```python
from build123d import *

# Parameters (mm, degrees)
SKETCH_1_W             = 56
SKETCH_1_H             = 54
EXTRUDE_492_DEPTH      = 12.5
SKETCH_3_W             = 36
SKETCH_3_H             = 46
CUT_EXTRUDE_735_DEPTH  = 41.856456038
SKETCH_11_R            = 1.25
CUT_EXTRUDE_988_DEPTH  = 10
CUT_EXTRUDE_1455_DEPTH = 8
CUT_EXTRUDE_1797_REACH = 65.413
SKETCH_4_R             = 4.2
SKETCH_6_R             = 4
CUT_EXTRUDE_1934_DEPTH = 10
SKETCH_7_W             = 6.25
SKETCH_7_H             = 20.5
CUT_EXTRUDE_2133_DEPTH = 10
SKETCH_8_R             = 5.25
CUT_EXTRUDE_2310_DEPTH = 2.25
SKETCH_9_R             = 0.75
CUT_EXTRUDE_2668_DEPTH = 4.75
CUT_EXTRUDE_3065_DEPTH = 41.856456038
CHAMFER_1_SIZE         = 1
FILLET_1_R             = 1
SKETCH_12_W            = 20
SKETCH_12_H            = 1.5
CUT_EXTRUDE_3477_DEPTH = 41.856456038
FILLET_2_R             = 0.5
CUT_EXTRUDE_4202_REACH = 42.856
SKETCH_13_W            = 36
SKETCH_13_H            = 5
EXTRUDE_4562_DEPTH     = 5
FILLET_3_R             = 10
FILLET_4_R             = 2
FILLET_6_R             = 1


with BuildPart() as part:
    # Эскиз1 → Extrude 492 (new body)
    with BuildSketch(Plane.XY):
        Rectangle(SKETCH_1_W, SKETCH_1_H)
    extrude(amount=EXTRUDE_492_DEPTH)

    # Эскиз3 → Cut-Extrude 735 (cut, through all)
    with BuildSketch(Plane.XY.offset(12.5)):
        with Locations((0, -1)):
            Rectangle(SKETCH_3_W, SKETCH_3_H)
    extrude(amount=-CUT_EXTRUDE_735_DEPTH, mode=Mode.SUBTRACT)

    # Эскиз11 → Cut-Extrude 988 (cut)
    with BuildSketch(Plane.XZ.offset(27)):
        with Locations(Location((-25, 5, 0), (0, 0, 270))):
            Circle(SKETCH_11_R)
        with Locations(Location((25, 5, 0), (0, 0, 270))):
            Circle(SKETCH_11_R)
    cut_extrude_988 = extrude(amount=-CUT_EXTRUDE_988_DEPTH, mode=Mode.SUBTRACT)

    # Mirror 1032: Cut-Extrude 988 across plane
    add(cut_extrude_988.mirror(Plane.ZX), mode=Mode.SUBTRACT)

    # Эскиз5 → Cut-Extrude 1455 (cut)
    with BuildSketch(Plane(origin=(28, 0, 0), x_dir=(0, 0, -1), z_dir=(1, 0, 0))):
        with BuildLine():
            Line((-9.688027281, -1.412461071), (-8.743079599, -14.085887362))
            ThreePointArc((-8.743079599, -14.085887362), (-6.25, -16.4), (-3.756920401, -14.085887362))
            Line((-3.756920401, -14.085887362), (-2.811972719, -1.412461071))
            ThreePointArc((-2.811972719, -1.412461071), (-6.25, 5.2), (-9.688027281, -1.412461071))
        make_face()
    extrude(amount=-CUT_EXTRUDE_1455_DEPTH, mode=Mode.SUBTRACT)

    # Эскиз4 → Cut-Extrude 1797 (cut, up to next)
    with BuildSketch(Plane(origin=(28, 0, 0), x_dir=(0, 0, -1), z_dir=(1, 0, 0)), mode=Mode.PRIVATE) as cut_extrude_1797_sk1:
        with Locations((-6.25, 1)):
            Circle(SKETCH_4_R)
    cut_extrude_1797_tool1 = extrude(cut_extrude_1797_sk1.sketch, amount=-CUT_EXTRUDE_1797_REACH, mode=Mode.PRIVATE) & part.part
    add(cut_extrude_1797_tool1.solids().sort_by_distance((28, 1, 6.25))[0], mode=Mode.SUBTRACT)

    # Эскиз6 → Cut-Extrude 1934 (cut)
    with BuildSketch(Plane.ZY.offset(28)):
        with Locations((6.25, 1)):
            Circle(SKETCH_6_R)
    extrude(amount=-CUT_EXTRUDE_1934_DEPTH, mode=Mode.SUBTRACT)

    # Эскиз7 → Cut-Extrude 2133 (cut)
    with BuildSketch(Plane.ZY.offset(28)):
        with Locations((9.375, 1)):
            Rectangle(SKETCH_7_W, SKETCH_7_H)
    extrude(amount=-CUT_EXTRUDE_2133_DEPTH, mode=Mode.SUBTRACT)

    # Эскиз8 → Cut-Extrude 2310 (cut, symmetric)
    with BuildSketch(Plane.ZY.offset(23)):
        with Locations((6.25, 1)):
            Circle(SKETCH_8_R)
    extrude(amount=CUT_EXTRUDE_2310_DEPTH, both=True, mode=Mode.SUBTRACT)

    # Эскиз9 → Cut-Extrude 2668 (cut)
    with BuildSketch(Plane.XY.offset(6.25)):
        with Locations((-23, 8)):
            Circle(SKETCH_9_R)
        with Locations((-23, -6)):
            Circle(SKETCH_9_R)
    extrude(amount=-CUT_EXTRUDE_2668_DEPTH, mode=Mode.SUBTRACT)

    # Эскиз10 → Cut-Extrude 3065 (cut, through all)
    with BuildSketch(Plane.XY.offset(12.5)):
        Polygon((28, -18.3), (28, 10.7), (22.5, 5.2), (22.5, -12.8), align=None)
    extrude(amount=-CUT_EXTRUDE_3065_DEPTH, mode=Mode.SUBTRACT)

    # Фаска1
    chamfer_1_edges = [part.edges().sort_by_distance(p)[0] for p in [
        (-28, 1, 2.25),
        (-18, 1, 2.25),
    ]]
    chamfer(chamfer_1_edges, length=CHAMFER_1_SIZE)

    # Скругление1
    fillet_1_edges = [part.edges().sort_by_distance(p)[0] for p in [
        (18, -24, 6.25),
        (-18, -24, 6.25),
    ]]
    fillet(fillet_1_edges, radius=FILLET_1_R)

    # Эскиз12 → Cut-Extrude 3477 (cut, through all)
    with BuildSketch(Plane.XY):
        with Locations((0, -24.75)):
            Rectangle(SKETCH_12_W, SKETCH_12_H)
    extrude(amount=CUT_EXTRUDE_3477_DEPTH, mode=Mode.SUBTRACT)

    # Скругление2
    fillet_2_edges = [part.edges().sort_by_distance(p)[0] for p in [
        (-10, -24, 6.25),
        (-10, -25.5, 6.25),
        (10, -25.5, 6.25),
        (10, -24, 6.25),
    ]]
    fillet(fillet_2_edges, radius=FILLET_2_R)

    # Эскиз13 → Cut-Extrude 4202 (cut, up to next)
    with BuildSketch(Plane.XY.offset(12.5), mode=Mode.PRIVATE) as cut_extrude_4202_sk1:
        with Locations((0, 24.5)):
            Rectangle(SKETCH_13_W, SKETCH_13_H)
    cut_extrude_4202_tool1 = extrude(cut_extrude_4202_sk1.sketch, amount=-CUT_EXTRUDE_4202_REACH, mode=Mode.PRIVATE) & part.part
    add(cut_extrude_4202_tool1.solids().sort_by_distance((0, 24.5, 12.5))[0], mode=Mode.SUBTRACT)

    # Эскиз14 → Extrude 4562 (add)
    with BuildSketch(Plane(origin=(0, 27, 0), x_dir=(1, 0, 0), z_dir=(0, 1, 0))):
        Polygon((-28, -12.5), (-28, -28), (28, -28), (28, -12.5), (18, -12.5), (18, -22.5), (-18, -22.5), (-18, -12.5), align=None)
    extrude(amount=-EXTRUDE_4562_DEPTH)

    # Скругление3
    fillet_3_edges = [part.edges().sort_by_distance(p)[0] for p in [
        (23, 22, 12.5),
        (-23, 22, 12.5),
    ]]
    fillet(fillet_3_edges, radius=FILLET_3_R)

    # Скругление4
    fillet_4_edges = [part.edges().sort_by_distance(p)[0] for p in [
        (0, 22, 22.5),
        (0, 22, 28),
        (-28, 24.5, 28),
        (0, 27, 28),
    ]]
    fillet(fillet_4_edges, radius=FILLET_4_R)

    # Скругление6
    fillet_6_edges = [part.edges().sort_by_distance(p)[0] for p in [
        (28, -22.65, 12.5),
    ]]
    fillet(fillet_6_edges, radius=FILLET_6_R)


solid = part.part
```
Work out the finished part from the listing and answer in its coordinate system (mm). A direction names the side the tool comes from. Round coordinates to 2 decimals unless told otherwise and drop trailing zeros. Write each loop counter-clockwise with the first axis right and the second up, starting at its lowest first coordinate (ties: lowest second). Pieces come first, ordered by that corner, then holes.
1) A cutting plane is placed at A-A on z = 14.5. Determine the outline of the cut face in (x, y).
2) Which of the six approach directions +Z, -Z, +X, -X, +Y, -Y give full straight-line access (tool end or side, diameter ignored) to faces 4 (the face through (-23, 9, 6.25)), 5 (the face through (-23, -6, 1.5)), 6 (the face through (0, 26, 22.5)), 7 (the face through (20, -9, 6)), 8 (the face through (0, -25.5, 6))?
3) A cutting plane is placed at C-C on y = 1. Determine the outline of the cut face in (x, z).
4) Determine the mould class of faces 1 (the face through (22.4, -16.4, 6.3)), 2 (the face through (22.93, 19.15, 15.51)), 3 (the face through (18, 8, 7)) for opening direction Y: pulls with the +Y half, pulls with the -Y half, needs draft (parallel to the pull), parting line crosses it, or undercut.
5) Flat-ended cylindrical pins translate along their axes: P1, Ø1.2, axis at x = -23, y = -6, coming from the +Z side; P2, Ø2, axis at x = -25, z = 5, coming from the +Y side; P3, Ø7, axis at y = -1.5, z = 2.5, coming from the +X side. Find the tip coordinate at first contact, or state that the pin passes through.
6) Consider probe 1 along X at (y, z) = (20.5, 5); probe 2 along X at (y, z) = (-20.5, 6.5); probe 3 along Y at (x, z) = (-3, 1.5). Determine where each line is inside the solid, lowest interval first.
7) A cutting plane is placed at B-B on x = 12.5. Determine the outline of the cut face in (y, z).
8) A cutting plane is placed at D-D on x = -21.5. Determine the outline of the cut face in (y, z), and give its area (3 significant figures).
Entries:
1. outline: (-28, 18) - (-18, 18) - (-18, 27) - (-28, 27) - close; (18, 18) - (28, 18) - (28, 27) - (18, 27) - close
2. face 4: +Z, -X
2. face 5: +Z
2. face 6: -Z, +Y, -Y
2. face 7: +X
2. face 8: +Z, -Z, +Y
3. outline: (-28, 0) - (-18, 0) - (-18, 1.25) - (-19, 2.25) - (-20.75, 2.25) - (-20.75, 1) - (-25.25, 1) - (-25.25, 2.25) - (-27, 2.25) - (-28, 1.25) - close; (18, 0) - (22.5, 0) - (22.5, 2.05) - (18, 2.05) - close; (18, 10.45) - (22.5, 10.45) - (22.5, 12.5) - (18, 12.5) - close
4. face 1: undercut
4. face 2: pulls with the -Y half
4. face 3: needs draft
5. P1: stops at z = 1.5
5. P2: stops at y = 17
5. P3: stops at x = 22.5
6. probe 1: x = -28 to -26.25, -23.75 to -18, 18 to 23.75, 26.25 to 28
6. probe 2: x = -28 to -18, 18 to 28
6. probe 3: y = -27 to -25.5
7. outline: (-27, 0) - (-24, 0) - (-24, 12.5) - (-27, 12.5) - close; (22, 24.5) arc R2 ccw to (24, 22.5) - (27, 22.5) - (27, 26) arc R2 ccw to (25, 28) - (24, 28) arc R2 ccw to (22, 26) - close
8. outline: (-27, 0) - (27, 0) - (27, 26) arc R2 ccw to (25, 28) - (24, 28) arc R2 ccw to (22, 26) - (22, 22.5) arc R10 cw to (12, 12.5) - (11.25, 12.5) - (11.25, 6.25) - (6.25, 6.25) arc R5.25 cw to (-4.25, 6.25) - (-9.25, 6.25) - (-9.25, 12.5) - (-27, 12.5) - close
8. area: 601 mm2
